Autodesk Inventor part; units mm, degrees
ref_plane "YZ Plane" through (0, 0, 0) normal (1, 0, 0) x (0, 1, 0)
ref_plane "XZ Plane" through (0, 0, 0) normal (0, 1, 0) x (-1, 0, 0)
ref_plane "XY Plane" through (0, 0, 0) normal (0, 0, 1) x (1, 0, 0)
sketch "Skizze1" plane through (0, 0, 0) normal (0, 0, 1) x (1, 0, 0)
  line L0 (-18.5, -9) -> (18.5, -9)
  line L1 (18.5, -9) -> (18.5, 9)
  line L2 (18.5, 9) -> (-18.5, 9)
  line L3 (-18.5, 9) -> (-18.5, -9)
  line L4 (-18.5, -9) -> (18.5, 9) construction
  line L5 (18.5, -9) -> (-18.5, 9) construction
  line L6 (-20.5, 11) -> (20.5, 11)
  line L7 (20.5, 11) -> (20.5, -11)
  line L8 (20.5, -11) -> (-20.5, -11)
  line L9 (-20.5, -11) -> (-20.5, 11)
  point P0 (0, 0)
  dimension "d0" = 18
  dimension "d1" = 37
  dimension "d2" = 2
extrude "Extrusion1" add sketch "Skizze1" against normal blind 1 contours L3 L2 L1 L0 | L6 L7 L8 L9
extrude "Extrusion2" add sketch "Skizze1" along normal blind 6
sketch "Skizze2" plane through (0, 0, 6) normal (0, 0, 1) x (1, 0, 0)
  line L0 (-18.5, -9) -> (-18.5, 9)
  line L1 (-18.5, 9) -> (18.5, 9)
  line L2 (18.5, 9) -> (18.5, -9)
  line L3 (18.5, -9) -> (-18.5, -9)
  line L4 (20.5, 11) -> (-20.5, 11)
  line L5 (-20.5, 11) -> (-20.5, -11)
  line L6 (-20.5, -11) -> (20.5, -11)
  line L7 (20.5, -11) -> (20.5, 11)
  line L8 (-20.5, -6) -> (0, -6)
  line L9 (0, -6) -> (0, 6)
  line L10 (0, 6) -> (-20.5, 6)
  line L11 (-20.5, 6) -> (-20.5, -6)
  line L12 (-20.5, 11) -> (-20.5, -11)
  point P0 (0, 0)
  point P1 (0, 0)
  dimension "d7" = 12
extrude "Extrusion3" cut sketch "Skizze2" against normal blind 5 contours L8 L5 L10 L0 | L0 L10 L9 L8
sketch "Skizze3" plane through (0, 0, 6) normal (0, 0, 1) x (1, 0, 0)
  line L0 (-20.5, 6) -> (-18.5, 6)
  line L1 (-18.5, 6) -> (-18.5, 9)
  line L2 (-18.5, 9) -> (18.5, 9)
  line L3 (18.5, 9) -> (18.5, -9)
  line L4 (18.5, -9) -> (-18.5, -9)
  line L5 (-18.5, -9) -> (-18.5, -6)
  line L6 (-18.5, -6) -> (-20.5, -6)
  line L7 (-20.5, -6) -> (-20.5, -11)
  line L8 (-20.5, -11) -> (20.5, -11)
  line L9 (20.5, -11) -> (20.5, 11)
  line L10 (20.5, 11) -> (-20.5, 11)
  line L11 (-20.5, 11) -> (-20.5, 6)
  line L12 (20.5, -4) -> (0, -4)
  line L13 (0, -4) -> (0, 4)
  line L14 (0, 4) -> (20.5, 4)
  line L15 (20.5, 4) -> (20.5, -4)
  point P0 (0, 0)
  point P1 (0, 0)
  point P2 (20.5, 0)
  dimension "d10" = 8
extrude "Extrusion4" cut sketch "Skizze3" against normal blind 5 contours L9 L12 L3 L14 | L3 L12 L13 L14
sketch "Skizze4" plane through (0, 0, 6) normal (0, 0, 1) x (1, 0, 0)
  line L0 (20.5, -4) -> (18.5, -4)
  line L1 (18.5, -4) -> (18.5, -9)
  line L2 (18.5, -9) -> (-18.5, -9)
  line L3 (-18.5, -9) -> (-18.5, -6)
  line L4 (-18.5, -6) -> (-20.5, -6)
  line L5 (-20.5, -6) -> (-20.5, -11)
  line L6 (-20.5, -11) -> (20.5, -11)
  line L7 (20.5, -11) -> (20.5, -4)
  line L8 (18.5, 4) -> (20.5, 4)
  line L9 (20.5, 4) -> (20.5, 11)
  line L10 (20.5, 11) -> (-20.5, 11)
  line L11 (-20.5, 11) -> (-20.5, 6)
  line L12 (-20.5, 6) -> (-18.5, 6)
  line L13 (-18.5, 6) -> (-18.5, 9)
  line L14 (-18.5, 9) -> (18.5, 9)
  line L15 (18.5, 9) -> (18.5, 4)
  point P0 (0, 0)
extrude "Extrusion5" add sketch "Skizze4" along normal blind 2
fillet "Rundung1" radius 1 4 edges at (20.5, 11, 3.5) (-20.5, 11, 3.5) (-20.5, -11, 3.5) (20.5, -11, 3.5)
properties part number "USB_case_A"
Build history of the part. All positions in model axes, mm. A direction names the side the tool comes from. Coordinates: 2 decimals unless noted, no trailing zeros. Order: outer loops, then holes, each group sorted by start corner. A loop starts at its lowest first (then second) coordinate and runs counter-clockwise, first axis right, second up. Notation, with made-up numbers: (82, 6.5) - (92, 6.5) arc R18 ccw to (92, 21.5) - close; hole circle Ø2 at (7, 44.5). An arc over 180 degrees is marked (long way). Write item = value, one per line. Start each with the question number.
1) Saw through at B-B on y = 0. Write the cut outline in (x, z).
2) Saw through at A-A on z = 1.75. Write the cut outline in (x, y), then the cut area to 3 significant figures.
3) Two-plate mould, pull along X, no slides. Class faces 1 (the face through (19, 4, 5)), 2 (the face through (0, 0, 0)), 3 (the face through (-18.5, -2.1, 0.4)), 4 (the face through (20.215, -10.699, 3.437)): pulls with the +X half, pulls with the -X half, needs draft (parallel to the pull), parting line crosses it, or undercut.
4) Flat gauge pins, fed straight in: pin 1 Ø1.5 at (x, y) = (-2, 1) entering from +Z; pin 2 Ø0.6 at (x, z) = (20, 3) entering from +Y; pin 3 Ø0.6 at (x, y) = (19, 1) entering from +Z. Where does each tip first touch, or does it go through?
5) Wall check: line 1 along Y through (x, z) = (-12, 1.5); line 2 along X through (y, z) = (3, 0.75); line 3 along Z through (x, y) = (-5, 7.5). Give the ranges that are in metal, low to high. Write a range as from..to.
6) Saw through at C-C on x = 3. Write the cut outline in (y, z), then the cut area to 3 significant figures.
7) 3-axis set-ups, long thin cutter, end or side, ignore diameter. For faces 5 (the face through (-20, 0, 1)), 6 (the face through (-20.215, -10.699, 3.563)), 7 (the face through (0, -9, 4)), 8 (the face through (20.5, 0, 0)), 9 (the face through (20, -4, 5)): which of +Z, -Z, +X, -X, +Y, -Y reach the whole face in a straight line?
From the geometry:
q1.outline = (-20.5, -1) - (20.5, -1) - (20.5, 1) - (18.5, 1) - (18.5, 0) - (-18.5, 0) - (-18.5, 1) - (-20.5, 1) - close
q2.outline = (-20.5, -10) arc R1 ccw to (-19.5, -11) - (19.5, -11) arc R1 ccw to (20.5, -10) - (20.5, -4) - (18.5, -4) - (18.5, -9) - (-18.5, -9) - (-18.5, -6) - (-20.5, -6) - close; (-20.5, 6) - (-18.5, 6) - (-18.5, 9) - (18.5, 9) - (18.5, 4) - (20.5, 4) - (20.5, 10) arc R1 ccw to (19.5, 11) - (-19.5, 11) arc R1 ccw to (-20.5, 10) - close
q2.area = 195 mm^2
q3.face_1 = needs draft
q3.face_2 = undercut
q3.face_3 = undercut
q3.face_4 = pulls with the +X half
q4.pin_1 = 0
q4.pin_2 = 10.98
q4.pin_3 = 1
q5.line_1 = -11..-9, 9..11
q5.line_2 = -20.5..-18.5, 18.5..20.5
q5.line_3 = -1..0
q6.outline = (-11, -1) - (11, -1) - (11, 8) - (9, 8) - (9, 0) - (-9, 0) - (-9, 8) - (-11, 8) - close
q6.area = 54.0 mm^2
q7.face_5 = +Z, -X
q7.face_6 = +Z, -Z, -X, -Y
q7.face_7 = +Z
q7.face_8 = +Z, -Z, +X, +Y, -Y
q7.face_9 = +Z, +X, -X
